Verification items for this drawing (mm, ordinates from the low corner). A direction names the side the tool comes from. Give positions to 0.01 mm unless a question says otherwise; leave off trailing zeros. Loops run counter-clockwise (first coordinate to the right, second up) from the corner with the lowest first, then second, coordinate; pieces in that order, holes last. Notation, with made-up numbers: M -31,78.5 L -19,78.5 A19 ccw -19,107.5 Z; hole C -33,-34 d1. An arc over 180 degrees is marked long. Use one line per item in the form item = value.
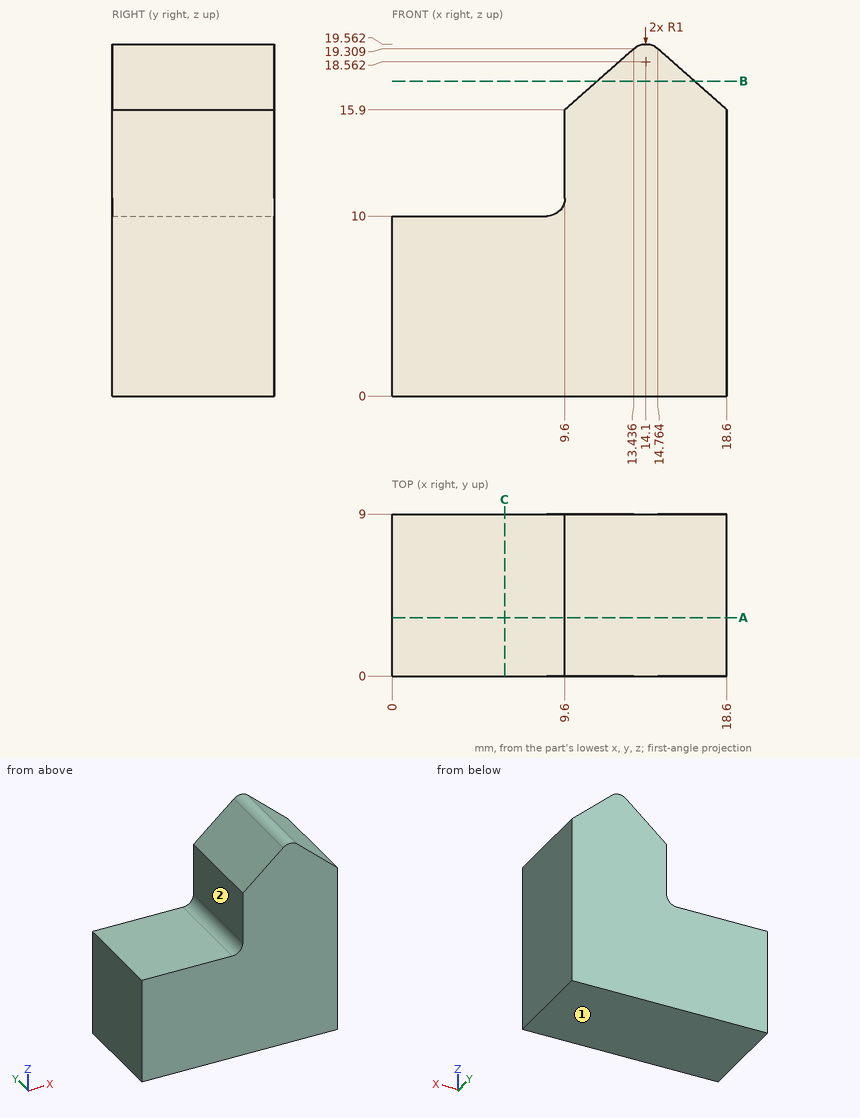
1) Section check A-A (y = 3.25). Record the cut outline in (x, z) (1 decimal).
Evaluation:
outline = M 0,0 L 18.6,0 L 18.6,15.9 L 14.8,19.3 A1 ccw 13.4,19.3 L 9.6,15.9 L 9.6,11 A1 cw 8.6,10 L 0,10 Z
2) Section check C-C (x = 6.25). Record the cut outline in (y, z).
Evaluation:
outline = M 0,0 L 9,0 L 9,10 L 0,10 Z
3) Scan lines: line 1 (Z direction, x = 7, y = 5); line 2 (X direction, y = 7, z = 14.75); line 3 (Z direction, x = 9.5, y = 5.5) (1 decimal). Record each from-to range of solid material in increasing order.
Evaluation:
line_1 = 0 to 10
line_2 = 9.6 to 18.6
line_3 = 0 to 10.6
4) Section check B-B (z = 17.5). Record the cut outline in (x, y).
Evaluation:
outline = M 11.4,0 L 16.8,0 L 16.8,9 L 11.4,9 Z
5) Depth check by flat-ended pin: pin 1 Ø2 at (y, z) = (1.5, 5.5) entering from -X; pin 2 Ø1.5 at (y, z) = (4, 13) entering from -X; pin 3 Ø3 at (x, y) = (11.5, 3.5) entering from +Z; pin 4 Ø2 at (x, y) = (16.5, 2) entering from +Z (1 decimal). Enter the tip coordinate at first touch or a pass-through.
Evaluation:
pin_1 = 0
pin_2 = 9.6
pin_3 = 18.92
pin_4 = 18.7
6) Set-up check for the marked faces 1 and 2: record each of +Z, -Z, +X, -X, +Y, -Y from which the full face is reachable in a straight line by a thin tool's end or side.
Evaluation:
face_1 = -Z, +X, -X, +Y, -Y
face_2 = +Z, -X, +Y, -Y
